Design review of the part built by this model. Coordinates are the model's own, in mm. Face numbers are marked on the shaded views. A direction names the side the tool comes from. Give positions to 0.01 mm unless a question says otherwise; leave off trailing zeros. Use CSV: the item, a comma, the result in double quotes.
```python
from build123d import *

# Parameters (mm, degrees)
PAD004_DEPTH    = 4
CHAMFER002_SIZE = 0.8
PAD015_DEPTH    = 4
SKETCH039_R     = 1.075
POCKET005_DEPTH = 10
FILLET003_R     = 0.8


with BuildPart() as part:
    # Sketch015 → AdditiveLoft001 section 0
    with BuildSketch(Plane.XY.offset(36)):
        Polygon((-15.9, 10.72), (15.9, 10.72), (15.9, -7.877957), (10.977437, -10.72), (-10.977437, -10.72), (-15.9, -7.877957), align=None)
    # Sketch016 → AdditiveLoft001 section 1
    with BuildSketch(Plane.XY.offset(40)):
        Polygon((-13.9, -6.723257), (-13.9, 10.72), (13.9, 10.72), (13.9, -6.723257), (10.441539, -8.72), (-10.441539, -8.72), align=None)
    loft()

    # Sketch017 → Pad004 (new body)
    with BuildSketch(Plane.XY.offset(36)):
        Polygon((-14.3, 7.42), (14.3, 7.42), (14.3, -6.838727), (10.521924, -9.02), (-10.521924, -9.02), (-14.3, -6.838727), align=None)
        Polygon((-11.1, 4.22), (11.1, 4.22), (11.1, -4.991206), (9.664486, -5.82), (-9.664486, -5.82), (-11.1, -4.991206), align=None, mode=Mode.SUBTRACT)
    extrude(amount=-PAD004_DEPTH)

    # Chamfer002
    chamfer002_edges = [part.edges().sort_by_distance(p)[0] for p in [
        (-14.3, 0.290637, 32),
        (-12.410962, -7.929363, 32),
        (0, -9.02, 32),
        (12.410962, -7.929363, 32),
        (14.3, 0.290637, 32),
        (0, 7.42, 32),
    ]]
    chamfer(chamfer002_edges, length=CHAMFER002_SIZE)

    # Sketch040 (on DatumPlane) → Pad015 (join, symmetric)
    with BuildSketch(Plane(origin=(-14.8, 0.311769, 0), x_dir=(-1, 0, 0), z_dir=(0, 1, 0))):
        Polygon((-29.6, 34.958579), (-29.1, 35.458579), (-29.1, 34.458579), align=None)
        Polygon((0, 34.958579), (-0.5, 35.458579), (-0.5, 34.458579), align=None)
    extrude(amount=PAD015_DEPTH, both=True)

    # Sketch018 → AdditiveLoft002 section 0
    with BuildSketch(Plane.XY.offset(36)):
        with BuildLine():
            add(Edge.make_bspline(
                [(-7.8, -1.12), (-7.8, 3.210127), (-12.675, 1.045064), (-17.55, -1.12), (-12.675, -3.285064), (-7.8, -5.450127), (-7.8, -1.12)],
                knots=[0, 0, 0, 2.094395, 2.094395, 4.18879, 4.18879, 6.283185, 6.283185, 6.283185], degree=2, weights=[1, 0.5, 1, 0.5, 1, 0.5, 1]))
        make_face()
    # Sketch019 → AdditiveLoft002 section 1
    with BuildSketch(Plane.XY.offset(32)):
        with BuildLine():
            add(Edge.make_bspline(
                [(-4.55, -1.12), (-4.55, 3.210127), (-9.425, 1.045064), (-14.3, -1.12), (-9.425, -3.285064), (-4.55, -5.450127), (-4.55, -1.12)],
                knots=[0, 0, 0, 2.094395, 2.094395, 4.18879, 4.18879, 6.283185, 6.283185, 6.283185], degree=2, weights=[1, 0.5, 1, 0.5, 1, 0.5, 1]))
        make_face()
    loft()

    # Sketch039 (on DatumPlane) → Pocket005 (cut)
    with BuildSketch(Plane(origin=(-4.55, -1.12, 32), x_dir=(0, -1, 0), z_dir=(-0.630593, 0, 0.776114))):
        with Locations((0, -2.522371)):
            Circle(SKETCH039_R)
    extrude(amount=POCKET005_DEPTH, mode=Mode.SUBTRACT)

    # Fillet003
    fillet003_edges = [part.edges().sort_by_distance(p)[0] for p in [
        (-7.799837, -0.045, 32),
    ]]
    fillet(fillet003_edges, radius=FILLET003_R)


solid = part.part
```
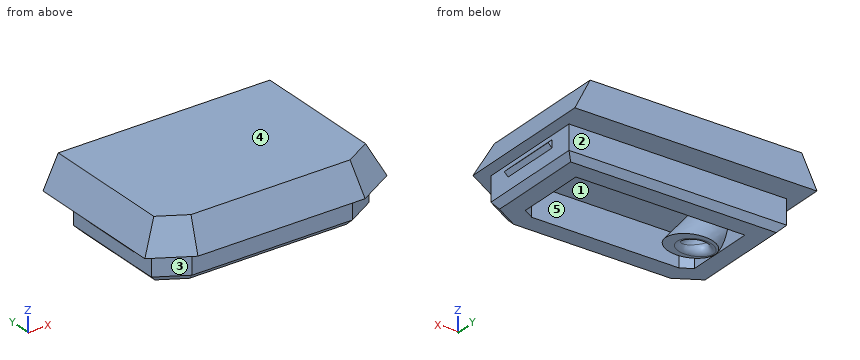
(1) Tool access review of the marked faces 4 and 5: name each direction out of +Z, -Z, +X, -X, +Y, -Y from which nothing blocks a thin tool from reaching the whole face with its end or side.
Established:
face 4,"+Z, +X, -X, +Y, -Y"
face 5,"-Z"
(2) Clearance check with flat-ended pins moving along their axes: pin 1 (4.5 mm diameter, centred on x = -0.5, z = 34, fed in from -Y); pin 2 (1.6 mm diameter, centred on y = 3.5, z = 35, fed in from +X); pin 3 (2.5 mm diameter, centred on x = 4.5, z = 34, fed in from +Y). State where each tip first meets the part, or that it passes through.
Established:
pin 1,"stops at y = -10.72"
pin 2,"stops at x = 14.8"
pin 3,"stops at y = 7.42"
(3) Mouldability with a two-part tool opening along Y and no side actions: class the marked faces 1, 2 and 3 as +Y half, -Y half, draft (parallel to the pull), parting line (faces both ways), or undercut.
Established:
face 1,"undercut"
face 2,"+Y half"
face 3,"-Y half"
(4) Take a section at A-A (z = 34). State how many separate pieces and enclosed holes the cut face has, then the cut area to 3 significant figures.
Established:
separate pieces,"1"
enclosed holes,"2"
area,"256 mm2"
(5) For line 1 along X through (y, z) = (-1.5, 33.75); line 2 along X through (y, z) = (-1, 34.25); line 3 along Y through (x, z) = (-10.5, 34.25), list the stretches that pass through material, from the lowest coordinate up. Write a range as [from, to].
Established:
line 1,"x = [-14.3, -10.52], [-7.93, -6.01], [11.1, 14.3]"
line 2,"x = [-14.3, -11], [-8.25, -6.38], [11.1, 14.3]"
line 3,"y = [-9.02, -5.34], [-3.53, -1.96], [-0.28, 1.29], [4.22, 7.42]"
